Input: part model. Units: mm. Frame: model coordinates. A direction names the side the tool comes from. Coordinates: 2 decimals unless noted, no trailing zeros. Order: outer loops, then holes, each group sorted by start corner. A loop starts at its lowest first (then second) coordinate and runs counter-clockwise, first axis right, second up. Notation, with made-up numbers: M 65,69 L 103,69 A18 cw 103,101 Z; hole C -16.5,-14.5 d6. An arc over 180 degrees is marked long. One line per item, written item: value.
```python
from build123d import *

# Parameters (mm, degrees)
F0_W     = 1117.6
F0_H     = 304.8
F0_W_2   = 9.525
F0_H_2   = 107.95
F1_DEPTH = 228.6
F0_W_3   = 320.675
F0_H_3   = 9.525
F0_W_4   = 254
F2_DEPTH = 228.6
F0_H_4   = 168.275
F3_DEPTH = 228.6
F4_DEPTH = 228.6
F5_DEPTH = 228.6


with BuildPart() as f1:
    # F0 (on Front) → F1 (new body)
    with BuildSketch(Plane.XZ):
        with Locations((43.0389853762, 152.4)):
            Rectangle(F0_W, F0_H)
        Polygon((-264.9360146238, 9.525), (-506.2360146238, 9.525), (-506.2360146238, 177.8), (-506.2360146238, 187.325), (-506.2360146238, 295.275), (-264.9360146238, 295.275), (-255.4110146238, 295.275), (65.2639853762, 295.275), (74.7889853762, 295.275), (328.7889853762, 295.275), (338.3139853762, 295.275), (592.3139853762, 295.275), (592.3139853762, 187.325), (592.3139853762, 177.8), (592.3139853762, 9.525), (338.3139853762, 9.525), (328.7889853762, 9.525), (74.7889853762, 9.525), (65.2639853762, 9.525), (-255.4110146238, 9.525), align=None, mode=Mode.SUBTRACT)
        Polygon((-506.2360146238, 187.325), (-506.2360146238, 177.8), (-264.9360146238, 177.8), (-264.9360146238, 9.525), (-255.4110146238, 9.525), (-255.4110146238, 177.8), (-255.4110146238, 187.325), (-264.9360146238, 187.325), align=None)
        with Locations((-260.1735146238, 241.3)):
            Rectangle(F0_W_2, F0_H_2)
    extrude(amount=F1_DEPTH)

    # F0 (on Front) → F2 (join, through all)
    with BuildSketch(Plane.XZ):
        with Locations((-95.0735146238, 182.5625)):
            Rectangle(F0_W_3, F0_H_3)
        with Locations((70.0264853762, 182.5625)):
            Rectangle(F0_W_2, F0_H_3)
        with Locations((201.7889853762, 182.5625)):
            Rectangle(F0_W_4, F0_H_3)
        with Locations((333.5514853762, 182.5625)):
            Rectangle(F0_W_2, F0_H_3)
        with Locations((465.3139853762, 182.5625)):
            Rectangle(F0_W_4, F0_H_3)
    extrude(amount=F2_DEPTH)

    # F0 (on Front) → F3 (join, through all)
    with BuildSketch(Plane.XZ):
        with Locations((333.5514853762, 93.6625)):
            Rectangle(F0_W_2, F0_H_4)
    extrude(amount=F3_DEPTH)

    # F0 (on Front) → F4 (join, through all)
    with BuildSketch(Plane.XZ):
        with Locations((-95.0735146238, 182.5625)):
            Rectangle(F0_W_3, F0_H_3)
        with Locations((70.0264853762, 93.6625)):
            Rectangle(F0_W_2, F0_H_4)
    extrude(amount=F4_DEPTH)

    # F0 (on Front) → F5 (join, through all)
    with BuildSketch(Plane.XZ):
        with Locations((70.0264853762, 241.3)):
            Rectangle(F0_W_2, F0_H_2)
        with Locations((333.5514853762, 241.3)):
            Rectangle(F0_W_2, F0_H_2)
    extrude(amount=F5_DEPTH)


solid = f1.part
```
(1) Draft query along Z for faces 1 (the flat face through (601.839, -113, 150)), 2 (the flat face through (204, -113, 9.525)), 3 (the flat face through (35, -113, 0)). Return one class per face: released by +Z, released by -Z, zero draft, split by the parting line, or undercut.
Data:
face 1: zero draft
face 2: undercut
face 3: released by -Z
(2) Cut plane B-B on z = 219. Output: boundary loops of the cut face in (x, y), plus the area to 3 significant figures.
Data:
outline: M -515.76,-228.6 L -506.24,-228.6 L -506.24,0 L -515.76,0 Z; M -264.94,-228.6 L -255.41,-228.6 L -255.41,0 L -264.94,0 Z; M 65.26,-228.6 L 74.79,-228.6 L 74.79,0 L 65.26,0 Z; M 328.79,-228.6 L 338.31,-228.6 L 338.31,0 L 328.79,0 Z; M 592.31,-228.6 L 601.84,-228.6 L 601.84,0 L 592.31,0 Z
area: 10,900 mm2
(3) Ray query, line 1 (X direction, y = -213, z = 35); line 2 (Z direction, x = -246, y = -162) (3 decimals). Return the intervals inside material, ascending. Write a range as from..to.
Data:
line 1: x = -515.76..-506.24, -264.94..-255.41, 65.26..74.79, 328.79..338.31, 592.31..601.84
line 2: z = 0..9.525, 177.8..187.325, 295.275..304.8
(4) Cut plane A-A on x = -48.5. Output: boundary loops of the cut face in (y, z) (3 decimals).
Data:
outline: M -228.6,0 L 0,0 L 0,9.525 L -228.6,9.525 Z; M -228.6,177.8 L 0,177.8 L 0,187.325 L -228.6,187.325 Z; M -228.6,295.275 L 0,295.275 L 0,304.8 L -228.6,304.8 Z
(5) Access query for faces 4 (the flat face through (592.314, -113, 95)), 5 (the flat face through (-515.761, -113, 150)). Directions: +Z, -Z, +X, -X, +Y, -Y. A direction counts if a zero-diameter tool reaches every point of the face in a straight line with its end or side. Return the directions, or none.
Data:
face 4: +Y, -Y
face 5: +Z, -Z, -X, +Y, -Y
(6) Cut plane C-C on y = -44. Give the number of separate pieces and of enclosed holes in the cut face, plus the area to 3 significant figures.
Data:
separate pieces: 1
enclosed holes: 8
area: 45,100 mm2
